```python
from build123d import *

# Parameters (mm, degrees)
F1_DEPTH = 131.318
F2_SIZE  = 33.02


with BuildPart() as f1:
    # F0 (on Top) → F1 (new body)
    with BuildSketch(Plane.XY):
        Polygon((-24.559464, -33.803202), (24.559464, -33.803202), (39.738047, 12.911674), (0, 41.783056), (-39.738047, 12.911674), align=None)
    extrude(amount=F1_DEPTH)

    # F2
    f2_edges = [f1.edges().sort_by_distance(p)[0] for p in [
        (0, -33.803202, 131.318),
        (-32.148756, -10.445764, 131.318),
        (-19.869024, 27.347365, 131.318),
        (19.869024, 27.347365, 131.318),
        (32.148756, -10.445764, 131.318),
    ]]
    chamfer(f2_edges, length=F2_SIZE)


solid = f1.part
```
Could you check a few things on this model? Use its own coordinates, in mm. Coordinates: 2 decimals unless noted, no trailing zeros. Loops run counter-clockwise (first coordinate to the right, second up) from the corner with the lowest first, then second, coordinate; pieces in that order, holes last.
1) Imagine slicing it at A-A (z = 33). List the corners of the cut face in (x, y) for me.
Reported:
outline: (-39.74, 12.91) - (-24.56, -33.8) - (24.56, -33.8) - (39.74, 12.91) - (0, 41.78) - close
2) Imagine slicing it at B-B (y = 7.5). List the corners of the cut face in (x, z) for me, and give its area (3 significant figures).
Reported:
outline: (-37.98, 0) - (37.98, 0) - (37.98, 98.3) - (23.08, 112.47) - (0, 126.03) - (-23.08, 112.47) - (-37.98, 98.3) - close
area: 8,640 mm2
3) Will these pins go through, and if not, where does the flat tip stop? pin 1 Ø4 at (x, y) = (21, -13) entering from +Z; pin 2 Ø8 at (x, z) = (14.5, 55) entering from +Y; pin 3 Ø4 at (x, y) = (-1.5, 8) entering from +Z.
Reported:
pin 1: stops at z = 110.11
pin 2: stops at y = 34.15
pin 3: stops at z = 126.75
4) Please list where these lines run through material, in increasing order: line 1 along X through (y, z) = (-23, 28); line 2 along Z through (x, y) = (-10.5, -1); line 3 along Z through (x, y) = (31, 9).
Reported:
line 1: x = -28.07 to 28.07
line 2: z = 0 to 121.81
line 3: z = 0 to 105.4
5) Imagine slicing it at C-C (x = 14.5). List the corners of the cut face in (y, z) for me, and give its area (3 significant figures).
Reported:
outline: (-33.8, 0) - (31.25, 0) - (31.25, 98.3) - (4.71, 119.77) - (-19.96, 112.14) - (-33.8, 98.3) - close
area: 7,210 mm2
6) Imagine slicing it at D-D (y = -28). List the corners of the cut face in (x, z) for me.
Reported:
outline: (-26.45, 0) - (26.45, 0) - (26.45, 98.3) - (20.34, 104.1) - (-20.34, 104.1) - (-26.45, 98.3) - close
